from build123d import *

# Parameters (mm, degrees)
BOSS_EXTRUDE1_DEPTH = 7
SKETCH2_W           = 10
SKETCH2_H           = 10
SKETCH2_W_2         = 5
BOSS_EXTRUDE2_DEPTH = 95
SKETCH15_R          = 1
CUT_EXTRUDE3_DEPTH  = 7
CIRPATTERN1_COUNT   = 8
CUT_EXTRUDE4_DEPTH  = 10
LPATTERN1_COUNT     = 8
LPATTERN1_PITCH     = 5.5


with BuildPart() as part:
    # Sketch1 → Boss-Extrude1 (new body)
    with BuildSketch(Plane(origin=(0, 0, 0), x_dir=(1, 0, 0), z_dir=(0, 1, 0))):
        with BuildLine():
            Line((-8, 56.940758688), (-8, 59.740758688))
            ThreePointArc((-8, 59.740758688), (-7.414213562, 61.154972251), (-6, 61.740758688))
            Line((-6, 61.740758688), (6, 61.740758688))
            ThreePointArc((6, 61.740758688), (7.414213562, 61.154972251), (8, 59.740758688))
            Line((8, 59.740758688), (8, 56.940758688))
            ThreePointArc((8, 56.940758688), (22.004297361, 53.123073119), (34.606342345, 45.920050844))
            Line((34.606342345, 45.920050844), (36.586241332, 47.899949831))
            ThreePointArc((36.586241332, 47.899949831), (38.000454895, 48.485736269), (39.414668457, 47.899949831))
            Line((39.414668457, 47.899949831), (47.899949831, 39.414668457))
            ThreePointArc((47.899949831, 39.414668457), (48.485736269, 38.000454895), (47.899949831, 36.586241332))
            Line((47.899949831, 36.586241332), (45.920050844, 34.606342345))
            ThreePointArc((45.920050844, 34.606342345), (53.123073119, 22.004297361), (56.940758688, 8))
            Line((56.940758688, 8), (59.740758688, 8))
            ThreePointArc((59.740758688, 8), (61.154972251, 7.414213562), (61.740758688, 6))
            Line((61.740758688, 6), (61.740758688, -6))
            ThreePointArc((61.740758688, -6), (61.154972251, -7.414213562), (59.740758688, -8))
            Line((59.740758688, -8), (56.940758688, -8))
            ThreePointArc((56.940758688, -8), (53.123073119, -22.004297361), (45.920050844, -34.606342345))
            Line((45.920050844, -34.606342345), (47.899949831, -36.586241332))
            ThreePointArc((47.899949831, -36.586241332), (48.485736269, -38.000454895), (47.899949831, -39.414668457))
            Line((47.899949831, -39.414668457), (39.414668457, -47.899949831))
            ThreePointArc((39.414668457, -47.899949831), (38.000454895, -48.485736269), (36.586241332, -47.899949831))
            Line((36.586241332, -47.899949831), (34.606342345, -45.920050844))
            ThreePointArc((34.606342345, -45.920050844), (22.004297361, -53.123073119), (8, -56.940758688))
            Line((8, -56.940758688), (8, -59.740758688))
            ThreePointArc((8, -59.740758688), (7.414213562, -61.154972251), (6, -61.740758688))
            Line((6, -61.740758688), (-6, -61.740758688))
            ThreePointArc((-6, -61.740758688), (-7.414213562, -61.154972251), (-8, -59.740758688))
            Line((-8, -59.740758688), (-8, -56.940758688))
            ThreePointArc((-8, -56.940758688), (-22.004297361, -53.123073119), (-34.606342345, -45.920050844))
            Line((-34.606342345, -45.920050844), (-36.586241332, -47.899949831))
            ThreePointArc((-36.586241332, -47.899949831), (-38.000454895, -48.485736269), (-39.414668457, -47.899949831))
            Line((-39.414668457, -47.899949831), (-47.899949831, -39.414668457))
            ThreePointArc((-47.899949831, -39.414668457), (-48.485736269, -38.000454895), (-47.899949831, -36.586241332))
            Line((-47.899949831, -36.586241332), (-45.920050844, -34.606342345))
            ThreePointArc((-45.920050844, -34.606342345), (-53.123073119, -22.004297361), (-56.940758688, -8))
            Line((-56.940758688, -8), (-59.740758688, -8))
            ThreePointArc((-59.740758688, -8), (-61.154972251, -7.414213562), (-61.740758688, -6))
            Line((-61.740758688, -6), (-61.740758688, 6))
            ThreePointArc((-61.740758688, 6), (-61.154972251, 7.414213562), (-59.740758688, 8))
            Line((-59.740758688, 8), (-56.940758688, 8))
            ThreePointArc((-56.940758688, 8), (-53.123073119, 22.004297361), (-45.920050844, 34.606342345))
            Line((-45.920050844, 34.606342345), (-47.899949831, 36.586241332))
            ThreePointArc((-47.899949831, 36.586241332), (-48.485736269, 38.000454895), (-47.899949831, 39.414668457))
            Line((-47.899949831, 39.414668457), (-39.414668457, 47.899949831))
            ThreePointArc((-39.414668457, 47.899949831), (-38.000454895, 48.485736269), (-36.586241332, 47.899949831))
            Line((-36.586241332, 47.899949831), (-34.606342345, 45.920050844))
            ThreePointArc((-34.606342345, 45.920050844), (-22.004297361, 53.123073119), (-8, 56.940758688))
        make_face()
    extrude(amount=BOSS_EXTRUDE1_DEPTH)

    # Sketch2 → Boss-Extrude2 (add)
    with BuildSketch(Plane(origin=(0, 7, 0), x_dir=(1, 0, 0), z_dir=(0, 1, 0))):
        with Locations((17, 10)):
            Rectangle(SKETCH2_W, SKETCH2_H)
        with Locations((-19.5, 10)):
            Rectangle(SKETCH2_W_2, SKETCH2_H)
    extrude(amount=BOSS_EXTRUDE2_DEPTH)

    # Sketch15 → Cut-Extrude3 (cut)
    with BuildSketch(Plane.XZ):
        with Locations(Location((0, 0, 0), (0, 0, 270))):
            Circle(SKETCH15_R)
    extrude(amount=-CUT_EXTRUDE3_DEPTH, mode=Mode.SUBTRACT)

    # Sketch16 → Cut-Loft2 section 0
    with BuildSketch(Plane.XZ):
        with BuildLine():
            Line((-6, 59.8), (6, 59.8))
            Line((6, 59.8), (6, 57.5))
            Line((6, 57.5), (-6, 57.5))
            Line((-6, 57.5), (-6, 59.8))
        make_face()
    # Sketch17 → Cut-Loft2 section 1
    with BuildSketch(Plane(origin=(0, 7, 0), x_dir=(1, 0, 0), z_dir=(0, 1, 0))):
        with BuildLine():
            Line((-6, -57.5), (6, -57.5))
            Line((6, -57.5), (6, -60.2))
            Line((6, -60.2), (-6, -60.2))
            Line((-6, -60.2), (-6, -57.5))
        make_face()
    cut_loft2 = loft(mode=Mode.SUBTRACT)

    # CirPattern1: Cut-Loft2 ×8 about axis
    cirpattern1_axis = Axis((0, 0, 0), (0, 1, 0))
    for i in range(1, CIRPATTERN1_COUNT):
        add(cut_loft2.rotate(cirpattern1_axis, i * 360 / CIRPATTERN1_COUNT), mode=Mode.SUBTRACT)

    # Sketch18 → Cut-Extrude4 (cut)
    with BuildSketch(Plane(origin=(0, 0, -15), x_dir=(-1, 0, 0), z_dir=(0, 0, -1))):
        Polygon((-12, 97.727940469), (-14, 97), (-14, 95), (-12, 94.272059531), align=None)
    cut_extrude4 = extrude(amount=-CUT_EXTRUDE4_DEPTH, mode=Mode.SUBTRACT)

    # LPattern1: Cut-Extrude4 ×8
    with Locations(*[(0, -i * LPATTERN1_PITCH, 0) for i in range(1, LPATTERN1_COUNT)]):
        add(cut_extrude4, mode=Mode.SUBTRACT)


solid = part.part
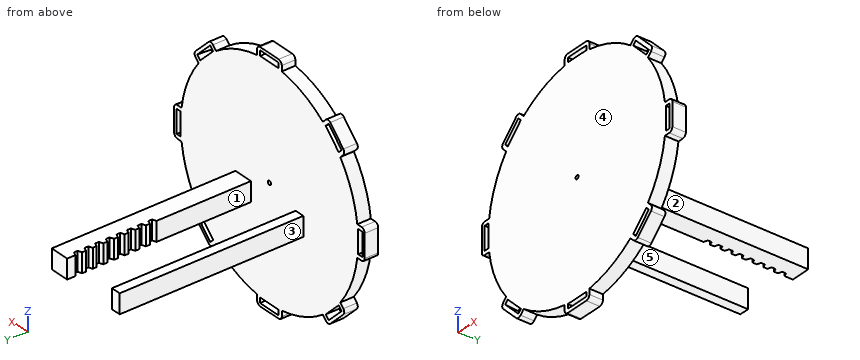
The model under review builds one solid part; all positions refer to its coordinate system, in mm. Face numbers are marked on the shaded views. A direction names the side the tool comes from. Give positions to 0.01 mm unless a question says otherwise; leave off trailing zeros. Order: outer loops, then holes, each group sorted by start corner. A loop starts at its lowest first (then second) coordinate and runs counter-clockwise, first axis right, second up. Notation, with made-up numbers: M 79,-0.5 L 114,-0.5 A24 cw 114,20.5 Z; hole C 4,84 d11. An arc over 180 degrees is marked long. One line per question, with ' | ' between items. Start each with the question number.
1) Consider section A-A, the plane z = -27. Give the boundary of the cut face in (x, y).
2) Consider section B-B, the plane z = 27.5. Give the boundary of the cut face in (x, y).
3) Clearance check with flat-ended pins moving along their axes: P1, Ø2, axis at y = 90.5, z = -12, coming from the -X side; P2, Ø2, axis at y = 3.5, z = -58.5, coming from the -X side; P3, Ø5, axis at y = 63, z = -11.5, coming from the +X side. State where each tip first meets the part, or that it passes through.
4) Wall thickness on L1, parallel to X at y = 11.5, z = -10.5; L2, parallel to X at y = 5.25, z = 0; L3, parallel to Y at x = -3, z = -25.5: over which ranges is each line inside the solid? List them lowest first. Write a range as from..to.
5) For the marked faces 4 and 5, list the 3-axis set-ups (+Z, -Z, +X, -X, +Y, -Y) from which the entire face can be reached by the end or side of a thin tool; tool diameter is ignored.
6) Mouldability with a two-part tool opening along X and no side actions: class the marked faces 1, 2 and 3 as pulls with the +X half, pulls with the -X half, needs draft (parallel to the pull), parting line crosses it, or undercut.
Found:
1) outline: M -50.77,0 L 50.77,0 L 50.77,7 L -50.77,7 Z
2) outline: M -50.5,0 L 50.5,0 L 50.5,7 L -50.5,7 Z
3) P1: stops at x = -22 | P2: stops at x = -8 | P3: stops at x = 22
4) L1: x = -22..-17, 12..22 | L2: x = -61.74..-60.1, -57.5..-1, 1..57.5, 60.1..61.74 | L3: y = 0..7
5) face 4: +Z, -Z, +X, -X, -Y | face 5: +Z, -Z, +Y
6) face 1: undercut | face 2: pulls with the +X half | face 3: pulls with the -X half
